Drawing for the job (mm, zero at the part's lowest x, y, z). A direction names the side the tool comes from. Give positions to 0.01 mm unless a question says otherwise; leave off trailing zeros. Write each loop counter-clockwise with the first axis right and the second up, starting at its lowest first coordinate (ties: lowest second). Pieces come first, ordered by that corner, then holes. Notation, with made-up numbers: M 22.25,35.5 L 58.25,35.5 A31 cw 58.25,68.5 Z; hole C 84.5,21 d9. An arc over 180 degrees is marked long. Use CSV: the item, a comma, the result in double quotes. Start each with the question number.
1. Band-saw the part on D-D, the plane y = 7.75. List the corners of the cut face in (x, z).
2. Drill centre lines: line 1 along Z through (x, y) = (33, 18.75); line 2 along Y through (x, z) = (4.5, 13). Where is each one in solid material? Low to high. Write a range as from..to.
3. Drop flat-ended pins along their axis: pin 1 Ø6 at (x, y) = (10.5, 19.5) entering from +Z; pin 2 Ø15 at (y, z) = (11.5, 15) entering from +X; pin 3 Ø1.5 at (x, y) = (24, 19.5) entering from -Z. Give the stop position or say it passes through.
4. Band-saw the part on C-C, the plane z = 12.25. List the corners of the cut face in (x, y), then the cut area to 3 significant figures.
5. Band-saw the part on B-B, the plane x = 5. List the corners of the cut face in (y, z).
6. Band-saw the part on A-A, the plane y = 12.7. List the corners of the cut face in (x, z).
7. 3-axis set-ups, long thin cutter, end or side, ignore diameter. For the marked faces 1 and 2: which of +Z, -Z, +X, -X, +Y, -Y reach the whole face in a straight line?
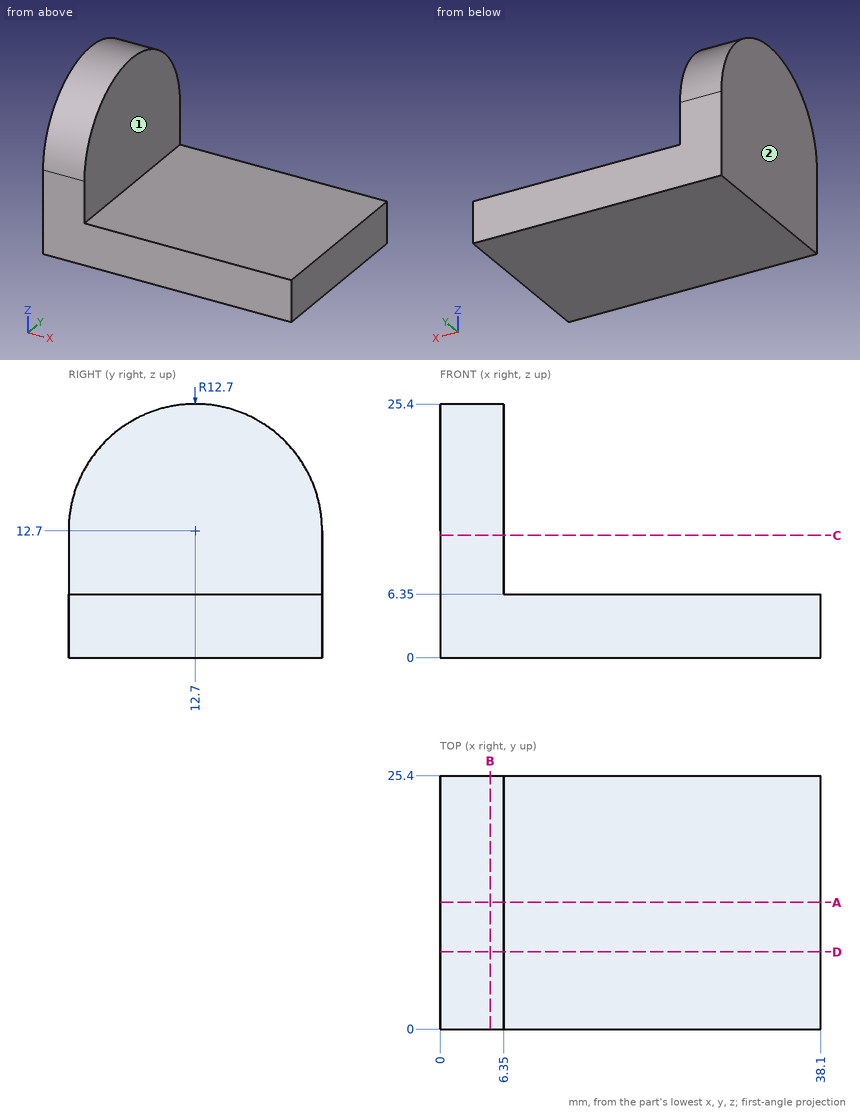
Output:
1,outline,"M 0,0 L 38.1,0 L 38.1,6.35 L 6.35,6.35 L 6.35,24.4 L 0,24.4 Z"
2,line 1,"z = 0..6.35"
2,line 2,"y = 0..25.4"
3,pin 1,"stops at z = 6.35"
3,pin 2,"stops at x = 6.35"
3,pin 3,"stops at z = 0"
4,outline,"M 0,0 L 6.35,0 L 6.35,25.4 L 0,25.4 Z"
4,area,"161 mm²"
5,outline,"M 0,0 L 25.4,0 L 25.4,12.7 A12.7 ccw 0,12.7 Z"
6,outline,"M 0,0 L 38.1,0 L 38.1,6.35 L 6.35,6.35 L 6.35,25.4 L 0,25.4 Z"
7,face 1,"+Z, +X, +Y, -Y"
7,face 2,"+Z, -Z, -X, +Y, -Y"
